For this review, take the finished solid that the model builds, in its own axes (mm). Face numbers are marked on the shaded views. A direction names the side the tool comes from. Round coordinates to 2 decimals unless told otherwise and drop trailing zeros. Loops run counter-clockwise (first coordinate to the right, second up) from the corner with the lowest first, then second, coordinate; pieces in that order, holes last.
1. Clearance check with flat-ended pins moving along their axes: pin 1 Ø4 at (x, y) = (7.5, -82) entering from -Z; pin 2 Ø6.5 at (x, y) = (0, -79.5) entering from +Z; pin 3 Ø10 at (x, z) = (14, 25.5) entering from +Y. State where each tip first meets the part, or that it passes through.
2. Consider section C-C on x = 15. State the section outline as (y, z) points, then the cut area to 3 significant figures.
3. To check wall thickness, follow line 1 along X through (y, z) = (-38, 19); line 2 along Y through (x, z) = (4.5, 23.5); line 3 along X through (y, z) = (-38, -6). State the ranges of each line that lie inside material, in increasing order.
4. Consider section D-D on y = 2. State the section outline as (x, z) points, then the cut area to 3 significant figures.
5. Draft analysis for pull direction X (two halves, no side actions). For the marked faces 1, 2 and 3, state which applies: released by +X, released by -X, zero draft, split by the parting line, or undercut.
6. Consider section A-A on y = -38.1. State the section outline as (x, z) points.
7. Consider section B-B on z = -22. State the section outline as (x, y) points.
8. Tool access review of the marked faces 4, 5, 6 and 7: name each direction out of +Z, -Z, +X, -X, +Y, -Y from which nothing blocks a thin tool from reaching the whole face with its end or side.
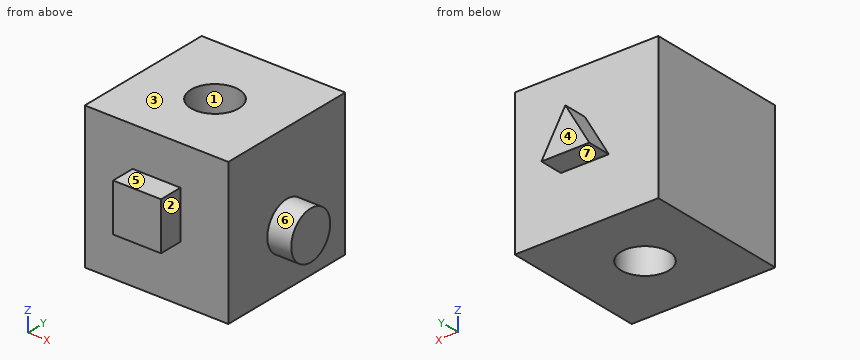
from build123d import *

# Parameters (mm, degrees)
F0_W      = 76.2
F0_H      = 76.2
F1_DEPTH  = 76.2
F3_D      = 25.4
F4_W      = 25.4
F4_H      = 25.4
F5_DEPTH  = 12.7
F6_R      = 12.7
F7_DEPTH  = 12.7
F5_FACE_W = 25.4
F5_FACE_H = 25.4
F9_DEPTH  = 12.7


with BuildPart() as f1:
    # F0 (on Front) → F1 (new body)
    with BuildSketch(Plane.XZ):
        with Locations((3.7895068526, 8.292155078)):
            Rectangle(F0_W, F0_H)
    extrude(amount=F1_DEPTH)

    # F3 (through all)
    with Locations(Plane.XY.offset(46.392155078)):
        with Locations((3.7895068526, -38.1)):
            Hole(F3_D / 2)

    # F4 (on face) → F5 (join)
    with BuildSketch(Plane.XZ.offset(76.2)):
        with Locations((3.7895068526, 12.7)):
            Rectangle(F4_W, F4_H)
    extrude(amount=F5_DEPTH)

    # F6 (on face) → F7 (join)
    with BuildSketch(Plane.YZ.offset(41.8895068526)):
        with Locations((-38.1, 0)):
            Circle(F6_R)
    extrude(amount=F7_DEPTH)

    # F8 (on face) + F5_face (on face) → F9 (join)
    with BuildSketch(Plane(origin=(0, 0, 0), x_dir=(-1, 0, 0), z_dir=(0, 1, 0))):
        Polygon((-17.3972853364, 0), (8.0027146636, 0), (-4.6972853364, 21.9970452561), align=None)
    with BuildSketch(Plane(origin=(3.7895068526, -88.9, 12.7), x_dir=(1, 0, 0), z_dir=(0, -1, 0))):
        Rectangle(F5_FACE_W, F5_FACE_H)
    extrude(amount=F9_DEPTH, dir=(0, 1, 0))


solid = f1.part
Resolved:
1. pin 1: stops at z = 0
1. pin 2: stops at z = 25.4
1. pin 3: stops at y = 0
2. outline: (-88.9, 0) - (-76.2, 0) - (-76.2, -29.81) - (-44.07, -29.81) - (-44.07, 46.39) - (-76.2, 46.39) - (-76.2, 25.4) - (-88.9, 25.4) - close; (-32.13, -29.81) - (0, -29.81) - (0, 0) - (12.7, 0) - (12.7, 4.15) - (0, 4.15) - (0, 46.39) - (-32.13, 46.39) - close
2. area: 5,270 mm2
3. line 1: x = -34.31 to -8.91, 16.49 to 41.89
3. line 2: y = -88.9 to -50.78, -25.42 to 0
3. line 3: x = -34.31 to -8.91, 16.49 to 54.59
4. outline: (-8, 0) - (17.4, 0) - (4.7, 22) - close
4. area: 279 mm2
5. face 1: undercut
5. face 2: released by +X
5. face 3: zero draft
6. outline: (-34.31, -29.81) - (-8.91, -29.81) - (-8.91, 46.39) - (-34.31, 46.39) - close; (16.49, -29.81) - (41.89, -29.81) - (41.89, -12.7) - (54.59, -12.7) - (54.59, 12.7) - (41.89, 12.7) - (41.89, 46.39) - (16.49, 46.39) - close
7. outline: (-34.31, -76.2) - (41.89, -76.2) - (41.89, 0) - (-34.31, 0) - close; hole circle Ø25.4 at (3.79, -38.1)
8. face 4: +Z, -Z, +X, -X, +Y
8. face 5: +Z, +X, -X, -Y
8. face 6: +X
8. face 7: -Z, +X, -X, +Y
